from build123d import *

# Parameters (mm, degrees)
BOSS_EXTRUDE1_DEPTH     = 7.9375
F_6_CLEARANCE_HOLE1_D   = 4.3053
CUT_EXTRUDE1_DEPTH      = 25.502197286
CUT_EXTRUDE1_DEPTH_BACK = 2.778125


with BuildPart() as part:
    # Sketch1 → Boss-Extrude1 (new body)
    with BuildSketch(Plane.XY):
        with BuildLine():
            Line((-19.05, 11.763375), (-19.05, 6.207125))
            Line((-19.05, 6.207125), (-13.350110486, 6.207125))
            ThreePointArc((-13.350110486, 6.207125), (-8.884072706, 4.37121478), (-7.000474108, -0.074920184))
            ThreePointArc((-7.000474108, -0.074920184), (-4.923806653, -4.976783982), (0, -7.000875))
            Line((0, -7.000875), (0, -3.825875))
            ThreePointArc((0, -3.825875), (-2.705302156, -2.705302156), (-3.825875, 0))
            Line((-3.825875, 0), (-3.825875, 11.763375))
            Line((-3.825875, 11.763375), (-19.05, 11.763375))
        make_face()
    extrude(amount=BOSS_EXTRUDE1_DEPTH)

    # #6 Clearance Hole1 (through all)
    with Locations(Plane(origin=(0, 11.763375, 0), x_dir=(1, 0, 0), z_dir=(0, 1, 0))):
        with Locations((-12.7, -3.96875)):
            Hole(F_6_CLEARANCE_HOLE1_D / 2)

    # Sketch4 → Cut-Extrude1 (cut, two sides: drawn at the far end of the back side and taken through both)
    with BuildSketch(Plane.XZ.offset(-6.207125).offset(-CUT_EXTRUDE1_DEPTH_BACK)):
        Polygon((-17.576011698, 3.96875), (-15.138005849, -0.254), (-10.261994151, -0.254), (-7.823988302, 3.96875), (-10.261994151, 8.1915), (-15.138005849, 8.1915), align=None)
    extrude(amount=CUT_EXTRUDE1_DEPTH + CUT_EXTRUDE1_DEPTH_BACK, mode=Mode.SUBTRACT)

    # Mirror1: part across plane


with BuildPart() as part_1:
    add(part.part)
    add(part.part.mirror(Plane(origin=(0, -3.825875, 7.9375), x_dir=(0, 0, 1), z_dir=(-1, 0, 0))))


solid = part_1.part
Geometry check sheet. Reference: the model listing, model coordinates, mm. A direction names the side the tool comes from. Give positions to 0.01 mm unless a question says otherwise; leave off trailing zeros. Order: outer loops, then holes, each group sorted by start corner. A loop starts at its lowest first (then second) coordinate and runs counter-clockwise, first axis right, second up.
1) Draft check along X on faces 1 (the cylindrical face through (7.544, 2.427, 3.913)), 2 (the flat face through (16.414, 7.616, 5.981)), 3 (the flat face through (-18, 6.207, 4)). Enter one of: released by +X, released by -X, zero draft, split by the parting line, or undercut.
Results are:
face 1: released by +X
face 2: undercut
face 3: zero draft
2) Gauge pin test, flat ends, axial feed: pin 1 (4 mm diameter, centred on x = 17, z = 4, fed in from -Y); pin 2 (2.5 mm diameter, centred on x = 11.5, z = 2.5, fed in from -Y). Record the tip position at first contact, or that the pin passes through.
Results are:
pin 1: stops at y = 6.21
pin 2: stops at y = 8.99
3) Cross-section at D-D (z = 7). Record the boundary of the cut face in (x, y), then the cut area to 3 significant figures.
Results are:
outline: (-19.05, 6.21) - (-15.83, 6.21) - (-15.83, 8.99) - (-9.57, 8.99) - (-9.57, 4.96) arc R6.35 cw to (-7, -0.07) arc R7 ccw to (7, -0.07) arc R6.35 cw to (9.57, 4.96) - (9.57, 8.99) - (15.83, 8.99) - (15.83, 6.21) - (19.05, 6.21) - (19.05, 11.76) - (3.83, 11.76) - (3.83, 0) arc R3.83 cw to (-3.83, 0) - (-3.83, 11.76) - (-19.05, 11.76) - close
area: 242 mm2
4) Cross-section at A-A (y = 7.5). Record the boundary of the cut face in (x, z).
Results are:
outline: (-19.05, 0) - (-15.28, 0) - (-17.58, 3.97) - (-15.28, 7.94) - (-19.05, 7.94) - close; (-10.12, 0) - (-3.83, 0) - (-3.83, 7.94) - (-10.12, 7.94) - (-7.82, 3.97) - close; (3.83, 0) - (10.12, 0) - (7.82, 3.97) - (10.12, 7.94) - (3.83, 7.94) - close; (15.28, 0) - (19.05, 0) - (19.05, 7.94) - (15.28, 7.94) - (17.58, 3.97) - close
5) Tool access check on faces 4 (the flat face through (18, 6.207, 4)), 5 (the flat face through (-10, 11.763, 4)), 6 (the flat face through (-3.826, 6, 4)), 7 (the flat face through (16.446, 7.616, 2.012)), 8 (the flat face through (5, 7, 0)). Record the directions out of +Z, -Z, +X, -X, +Y, -Y that give a thin tool (end or side, any length) a straight path to the whole face; none if there is none.
Results are:
face 4: +Z, -Z, +X, -Y
face 5: +Z, -Z, +X, -X, +Y
face 6: +Z, -Z, +Y
face 7: -Y
face 8: -Z, +X, -X, +Y, -Y
6) Cross-section at B-B (x = -12.7). Record the boundary of the cut face in (y, z).
Results are:
outline: (8.99, 0) - (11.76, 0) - (11.76, 1.82) - (8.99, 1.82) - close; (8.99, 6.12) - (11.76, 6.12) - (11.76, 7.94) - (8.99, 7.94) - close
7) Material ranges on probe 1 along Z at (x, y) = (-12.7, 9.6); probe 2 along X at (y, z) = (8.75, 5.5); probe 3 along Y at (x, z) = (17.5, 4.25), recorded low to high.
Results are:
probe 1: z = 0 to 1.82, 6.12 to 7.94
probe 2: x = -19.05 to -16.69, -8.71 to -3.83, 3.83 to 8.71, 16.69 to 19.05
probe 3: y = 6.21 to 11.76
8) Cross-section at C-C (z = 5). Record the boundary of the cut face in (x, y).
Results are:
outline: (-19.05, 6.21) - (-16.98, 6.21) - (-16.98, 8.99) - (-14.59, 8.99) - (-14.59, 11.76) - (-19.05, 11.76) - close; (-10.81, 8.99) - (-8.42, 8.99) - (-8.42, 3.86) arc R6.35 cw to (-7, -0.07) arc R7 ccw to (7, -0.07) arc R6.35 cw to (8.42, 3.86) - (8.42, 8.99) - (10.81, 8.99) - (10.81, 11.76) - (3.83, 11.76) - (3.83, 0) arc R3.83 cw to (-3.83, 0) - (-3.83, 11.76) - (-10.81, 11.76) - close; (14.59, 8.99) - (16.98, 8.99) - (16.98, 6.21) - (19.05, 6.21) - (19.05, 11.76) - (14.59, 11.76) - close
